Could you check a few things on this model? Use its own coordinates, in mm. A direction names the side the tool comes from. Coordinates: 2 decimals unless noted, no trailing zeros. Loops run counter-clockwise (first coordinate to the right, second up) from the corner with the lowest first, then second, coordinate; pieces in that order, holes last. Notation, with made-up numbers: (-36.75, 56) - (-4.75, 56) arc R22 ccw to (-4.75, 91) - close; hole circle Ø9 at (38.5, 34.25). An arc over 180 degrees is marked (long way). One line per item, written item: value. Start each with the question number.
(1) If I drill on line 1 along X through (y, z) = (32.5, 13.5); line 2 along Y through (x, z) = (-44, 9.5); line 3 along Y through (x, z) = (44, 8.5), over which ranges is the centre line in solid material (lowest first)? Write a range as from..to.
(2) If we section it at A-A on z = 1.5: Write out the boundary of the cut face in (x, y).
(3) If we section it at D-D on z = 13.75: Count the separate pieces of the cut face and the enclosed holes in it, then the cut area to 3 significant figures.
(4) I'm going to push flat-ended pins straight in: P1, Ø6, axis at x = 44, y = 32.5, coming from the -Z side; P2, Ø7, axis at x = 44.5, y = 10, coming from the -Z side. Where does each tip first touch, or does it pass through?
(5) If we section it at C-C on y = 32.5: Write out the boundary of the cut face in (x, z).
(6) On a 3-axis mill with a long thin cutter (end or side, diameter ignored), from which of +Z, -Z, +X, -X, +Y, -Y can I reach the whole of each face in a straight line? I mean faces 1 (the face through (51.75, 8, 7)), 2 (the face through (-1, 26.25, 13)), 3 (the face through (1, 51.25, 9)). Say none if no direction works.
(7) If we section it at B-B on x = 37: Write out the boundary of the cut face in (y, z).
(8) If we mould it in two halves opening along X, with no side actions, what happens to faces 4 (the face through (-4, -38, 0)), 5 (the face through (-39.75, 0, 11)), 6 (the face through (49.611, 58.995, 7.605))? For each: pulls with the +X half, pulls with the -X half, needs draft (parallel to the pull), parting line crosses it, or undercut.
```python
from build123d import *

# Parameters (mm, degrees)
F0_R     = 2.25
F0_W     = 79.5
F0_H     = 52.5
F1_DEPTH = 15
F2_W     = 8.5
F2_H     = 42.5
F2_W_2   = 71.5
F2_H_2   = 25
F3_DEPTH = 11
F4_W     = 96
F4_H     = 90
F5_DEPTH = 8
F6_R     = 7.5
F6_R_2   = 3.5
F6_R_3   = 5
F7_DEPTH = 15.001
F8_R     = 7.5


with BuildPart() as f1:
    # F0 (on Top) → F1 (new body)
    with BuildSketch(Plane.XY):
        Polygon((-51.75, -9.25), (-51.75, -44.25), (51.75, -44.25), (51.75, 61.25), (11.75, 61.25), (-3.25, 61.25), (-51.75, 61.25), align=None)
        with Locations((-44, -32.5)):
            Circle(F0_R, mode=Mode.SUBTRACT)
        with Locations((44, -32.5)):
            Circle(F0_R, mode=Mode.SUBTRACT)
        Rectangle(F0_W, F0_H, mode=Mode.SUBTRACT)
        with Locations((-44, 32.5)):
            Circle(F0_R, mode=Mode.SUBTRACT)
        with Locations((44, 32.5)):
            Circle(F0_R, mode=Mode.SUBTRACT)
    extrude(amount=F1_DEPTH)

    # F2 (on face) → F3 (cut)
    with BuildSketch(Plane(origin=(0, 0, 0), x_dir=(1, 0, 0), z_dir=(0, 0, -1))):
        with Locations((44, 0)):
            Rectangle(F2_W, F2_H)
        with Locations((0, -38.75)):
            Rectangle(F2_W_2, F2_H_2)
    extrude(amount=-F3_DEPTH, mode=Mode.SUBTRACT)

    # F4 (on face) → F5 (cut)
    with BuildSketch(Plane(origin=(0, 0, 0), x_dir=(1, 0, 0), z_dir=(0, 0, -1))):
        with Locations((-0.25, -8.25)):
            Rectangle(F4_W, F4_H)
    extrude(amount=-F5_DEPTH, mode=Mode.SUBTRACT)

    # F6 (on face) → F7 (cut, through all)
    with BuildSketch(Plane.XY.offset(15)):
        with Locations((-36.025, 44.25)):
            Circle(F6_R)
        with Locations((-4.275, 44.25)):
            Circle(F6_R_2)
        with Locations((37, 41.25)):
            Circle(F6_R_3)
    extrude(amount=-F7_DEPTH, mode=Mode.SUBTRACT)

    # F8
    f8_edges = [f1.edges().sort_by_distance(p)[0] for p in [
        (51.75, -44.25, 7.5),
        (-51.75, 61.25, 7.5),
        (-51.75, -44.25, 7.5),
        (51.75, 61.25, 7.5),
    ]]
    fillet(f8_edges, radius=F8_R)


solid = f1.part
```
Values:
1. line 1: x = -51.75..-46.25, -41.75..41.75, 46.25..51.75
1. line 2: y = -44.25..-34.75, -30.25..30.25, 34.75..61.25
1. line 3: y = -44.25..-34.75, -30.25..-21.25, 21.25..30.25, 34.75..61.25
2. outline: (-51.75, -36.75) arc R7.5 ccw to (-44.25, -44.25) - (44.25, -44.25) arc R7.5 ccw to (51.75, -36.75) - (51.75, 53.75) arc R7.5 ccw to (44.25, 61.25) - (-44.25, 61.25) arc R7.5 ccw to (-51.75, 53.75) - close; hole (-48.25, -36.75) - (47.75, -36.75) - (47.75, -21.25) - (48.25, -21.25) - (48.25, 21.25) - (47.75, 21.25) - (47.75, 53.25) - (-48.25, 53.25) - close
3. separate pieces: 1
3. enclosed holes: 8
3. area: 6,340 mm2
4. P1: stops at z = 8
4. P2: stops at z = 11
5. outline: (-51.75, 0) - (-48.25, 0) - (-48.25, 8) - (-46.25, 8) - (-46.25, 15) - (-51.75, 15) - close; (-41.75, 8) - (-35.75, 8) - (-35.75, 11) - (35.75, 11) - (35.75, 8) - (41.75, 8) - (41.75, 15) - (-41.75, 15) - close; (46.25, 8) - (47.75, 8) - (47.75, 0) - (51.75, 0) - (51.75, 15) - (46.25, 15) - close
6. face 1: +Z, -Z, +X, +Y, -Y
6. face 2: +Z, -Z
6. face 3: -Z
7. outline: (-44.25, 0) - (-36.75, 0) - (-36.75, 8) - (-26.25, 8) - (-26.25, 15) - (-44.25, 15) - close; (26.25, 8) - (36.25, 8) - (36.25, 15) - (26.25, 15) - close; (46.25, 8) - (53.25, 8) - (53.25, 0) - (61.25, 0) - (61.25, 15) - (46.25, 15) - close
8. face 4: needs draft
8. face 5: undercut
8. face 6: pulls with the +X half
